from build123d import *


with BuildPart() as part:
    # Эскиз22 → Revolve 1889 (revolve)
    with BuildSketch(Plane.XY):
        with BuildLine():
            Line((0.5, -2.8), (-0.3, -2.8))
            Line((-0.3, -2.8), (0.2, -3.3))
            Line((0.2, -3.3), (0.2, -4.25))
            Line((0.2, -4.25), (-3.4, -4.25))
            Line((-3.4, -4.25), (-3.8, -3.85))
            Line((-3.8, -3.85), (-3.8, -2.5))
            Line((-3.8, -2.5), (-3.511324865, -2))
            Line((-3.511324865, -2), (0.026794919, -2))
            Line((0.026794919, -2), (0.2, -2.3))
            Line((0.2, -2.3), (0.5, -2.3))
            ThreePointArc((0.5, -2.3), (0.691341716, -2.338060234), (0.853553391, -2.446446609))
            Line((0.853553391, -2.446446609), (2, -3.592893219))
            Line((2, -3.592893219), (2, -3.875735931))
            Line((2, -3.875735931), (1.787867966, -4.087867966))
            Line((1.787867966, -4.087867966), (0.5, -2.8))
        make_face()
    revolve(axis=Axis((0, 0, 0), (1, 0, 0)))


solid = part.part
Could you check a few things on this model? Use its own coordinates, in mm. A direction names the side the tool comes from. Coordinates: 2 decimals unless noted, no trailing zeros. Write each loop counter-clockwise with the first axis right and the second up, starting at its lowest first coordinate (ties: lowest second). Pieces come first, ordered by that corner, then holes. Notation, with made-up numbers: M 10,-25.75 L 33,-25.75 A8 ccw 33,-18.75 Z; hole C 59,48.25 d7. An arc over 180 degrees is marked long. One line per question, with ' | ' between items.
1) For pin 1 Ø1.5 at (x, z) = (-0.5, 2) entering from +Y; pin 2 Ø3 at (x, y) = (-1, -2) entering from -Z; pin 3 Ø1.5 at (x, y) = (0, -2.5) entering from +Z, each with a flat end and sliding along its axis, tell me the tip position at first contact or that it passes through.
Checks:
pin 1: y = 4.06 | pin 2: z = -4.22 | pin 3: z = 3.87
2) For faces 4 (the face through (-2, 0, 2)), 5 (the face through (0.1, 2.8, -0.1)), which set-ups out of +Z, -Z, +X, -X, +Y, -Y let a thin tool reach every point of the face, with its end or its side?
Checks:
face 4: +X, -X | face 5: none
3) I need wall thicknesses on probe 1 along Z at (x, y) = (0.35, 0); probe 2 along Y at (x, z) = (-0.9, 0). Which ranges of each line are inside material? Lowest first, please. Write a range as [from, to].
Checks:
probe 1: [-2.8, -2.3], [2.3, 2.8] | probe 2: [-4.25, -2], [2, 4.25]
4) Imagine slicing it at C-C, the plane x = -3.25. Write out the boundary of the cut face in (y, z), and give its area (3 significant figures).
Checks:
outline: C 0,0 d8.5; hole C 0,0 d4 | area: 44.2 mm²
5) Imagine slicing it at D-D, the plane x = 0.35. Write out the boundary of the cut face in (y, z).
Checks:
outline: C 0,0 d5.6; hole C 0,0 d4.6
6) If we mould it in two halves opening along Y, with no side actions, what happens to faces 1 (the face through (0.2, 2, 3)), 2 (the face through (0.35, 1.7, -1.55)), 3 (the face through (-1.625, -2.285, -3.584))? For each: released by +Y, released by -Y, zero draft, split by the parting line, or undercut.
Checks:
face 1: zero draft | face 2: undercut | face 3: split by the parting line
